```python
from build123d import *
from OCP.BRepFilletAPI import BRepFilletAPI_MakeChamfer

# Parameters (mm, degrees)
SKETCH_1_W          = 8
SKETCH_1_H          = 1
SKETCH_1_H_2        = 1.8
EXTRUDE_1_DEPTH     = 5.7
FILLET_1_R          = 0.8
CHAMFER_1_SIZE      = 0.5
CHAMFER_1_SIZE2     = 1.37373871
SKETCH_2_W          = 4.700894011
SKETCH_2_H          = 0.61177093
CUT_EXTRUDE_1_DEPTH = 5


with BuildPart() as part:
    # Эскиз1 → Бобышка-Вытянуть1 (new body)
    with BuildSketch(Plane.XY):
        with Locations((-3.289153283, 2.3)):
            Rectangle(SKETCH_1_W, SKETCH_1_H)
        with Locations((-3.289153283, 0.9)):
            Rectangle(SKETCH_1_W, SKETCH_1_H_2)
    extrude(amount=EXTRUDE_1_DEPTH)

    # Скругление1
    fillet_1_edges = [part.edges().sort_by_distance(p)[0] for p in [
        (0.710846717, 2.8, 2.85),
        (-7.289153283, 2.8, 2.85),
    ]]
    fillet(fillet_1_edges, radius=FILLET_1_R)

    # Фаска1: one chamfer whose edges measure the first distance from different faces: ONE call of the kernel's chamfer builder (chamfer() names one face for all edges)
    chamfer_1_edges_1 = [part.edges().sort_by_distance(p)[0] for p in [
        (0.710846717, 0, 2.85),
    ]]
    chamfer_1_side_1 = [part.faces().sort_by_distance(p)[0] for p in [
        (0.710846717, 1, 2.85),
    ]]
    chamfer_1_edges_2 = [part.edges().sort_by_distance(p)[0] for p in [
        (-7.289153283, 0, 2.85),
    ]]
    chamfer_1_side_2 = [part.faces().sort_by_distance(p)[0] for p in [
        (-7.289153283, 1, 2.85),
    ]]
    chamfer_1 = BRepFilletAPI_MakeChamfer(part.part.solid().wrapped)
    for e in chamfer_1_edges_1:
        chamfer_1.Add(CHAMFER_1_SIZE, CHAMFER_1_SIZE2, e.wrapped, chamfer_1_side_1[0].wrapped)  # the first distance lies on this face
    for e in chamfer_1_edges_2:
        chamfer_1.Add(CHAMFER_1_SIZE, CHAMFER_1_SIZE2, e.wrapped, chamfer_1_side_2[0].wrapped)  # the first distance lies on this face
    add(Compound.cast(chamfer_1.Shape()), mode=Mode.REPLACE)

    # Эскиз2 → Вырез-Вытянуть1 (cut)
    with BuildSketch(Plane(origin=(0, 0, 0), x_dir=(-1, 0, 0), z_dir=(0, 0, -1))):
        with BuildLine():
            Line((-0.310846717, 2), (-0.310846717, 0.780083015))
            Line((-0.310846717, 0.780083015), (0.733422785, 0.4))
            Line((0.733422785, 0.4), (5.844883781, 0.4))
            Line((5.844883781, 0.4), (6.889153283, 0.780083015))
            Line((6.889153283, 0.780083015), (6.889153283, 2))
            ThreePointArc((6.889153283, 2), (6.771995996, 2.282842712), (6.489153283, 2.4))
            Line((6.489153283, 2.4), (0.089153283, 2.4))
            ThreePointArc((0.089153283, 2.4), (-0.193689429, 2.282842712), (-0.310846717, 2))
        make_face()
        with Locations((3.494436776, 1.42533527)):
            Rectangle(SKETCH_2_W, SKETCH_2_H, mode=Mode.SUBTRACT)
    extrude(amount=-CUT_EXTRUDE_1_DEPTH, mode=Mode.SUBTRACT)


solid = part.part
```
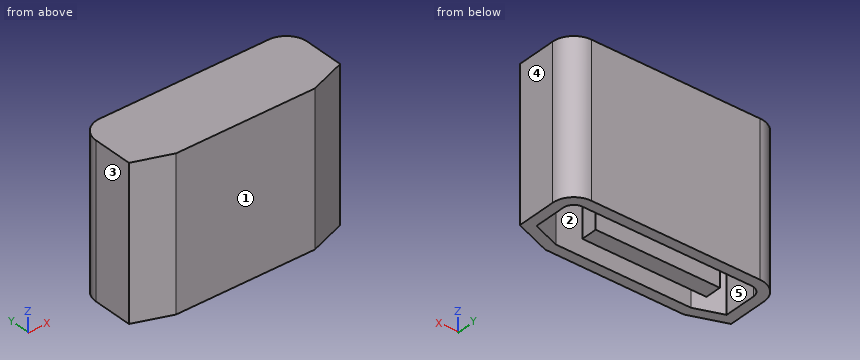
Input: part model. Units: mm. Frame: model coordinates. Face numbers are marked on the shaded views. A direction names the side the tool comes from. Round coordinates to 2 decimals unless told otherwise and drop trailing zeros. Order: outer loops, then holes, each group sorted by start corner. A loop starts at its lowest first (then second) coordinate and runs counter-clockwise, first axis right, second up. Notation, with made-up numbers: (-22.75, 84) - (31.25, 84) arc R12 cw to (31.25, 89) - close; hole circle Ø10 at (-4, 61). An arc over 180 degrees is marked (long way). Answer in a Markdown table with one row per item.
Item 1: Section query D-D (y = 1.55). Return the cut outline in (x, z).
Model answer:
| item | result |
|---|---|
| outline | (-7.29, 0) - (-6.89, 0) - (-6.89, 5) - (-5.84, 5) - (-5.84, 0) - (-1.14, 0) - (-1.14, 5) - (0.31, 5) - (0.31, 0) - (0.71, 0) - (0.71, 5.7) - (-7.29, 5.7) - close |
Item 2: Line query: line 1 (X direction, y = 1.6, z = 4.35); line 2 (Y direction, x = -3, z = 4.4); line 3 (X direction, y = 1.85, z = 0.8). Output: solid intervals per line, ascending.
Model answer:
| item | result |
|---|---|
| line 1 | x = -7.29 to -6.89, -5.84 to -1.14, 0.31 to 0.71 |
| line 2 | y = 0 to 0.4, 1.12 to 1.73, 2.4 to 2.8 |
| line 3 | x = -7.29 to -6.89, 0.31 to 0.71 |
Item 3: Section query C-C (x = -3.75). Return the cut outline in (y, z), then the cut area to 3 significant figures.
Model answer:
| item | result |
|---|---|
| outline | (0, 0) - (0.4, 0) - (0.4, 5) - (1.12, 5) - (1.12, 0) - (1.73, 0) - (1.73, 5) - (2.4, 5) - (2.4, 0) - (2.8, 0) - (2.8, 5.7) - (0, 5.7) - close |
| area | 9.02 mm² |
Item 4: Reachability of the marked faces 4 and 5 from +Z, -Z, +X, -X, +Y, -Y: full face, straight path, thin tool, end or side. Return the list, or none.
Model answer:
| item | result |
|---|---|
| face 4 | +Z, -Z, +X, +Y, -Y |
| face 5 | -Z |
Item 5: Section query B-B (y = 0.9). Return the cut outline in (x, z).
Model answer:
| item | result |
|---|---|
| outline | (-7.29, 0) - (-6.89, 0) - (-6.89, 5) - (0.31, 5) - (0.31, 0) - (0.71, 0) - (0.71, 5.7) - (-7.29, 5.7) - close |
Item 6: Section query A-A (z = 4.05). Return the cut outline in (x, y), then the cut area to 3 significant figures.
Model answer:
| item | result |
|---|---|
| outline | (-7.29, 0.5) - (-5.92, 0) - (-0.66, 0) - (0.71, 0.5) - (0.71, 2) arc R0.8 ccw to (-0.09, 2.8) - (-6.49, 2.8) arc R0.8 ccw to (-7.29, 2) - close; (-5.84, 1.12) - (-1.14, 1.12) - (-1.14, 1.73) - (-5.84, 1.73) - close; hole (-6.89, 0.78) - (-5.84, 0.4) - (-0.73, 0.4) - (0.31, 0.78) - (0.31, 2) arc R0.4 ccw to (-0.09, 2.4) - (-6.49, 2.4) arc R0.4 ccw to (-6.89, 2) - close |
| area | 10.4 mm² |
Item 7: Pin query (flat end, axial travel): pin 1 (1.5 mm diameter, centred on x = 0, z = 1.5, fed in from +Y). Return the tip coordinate at first contact, or that it passes through.
Model answer:
| item | result |
|---|---|
| pin 1 | stops at y = 2.8 |
Item 8: Mould query, pull axis Y, two halves, no side actions, for the marked faces 1, 2 and 3. Classes: released by +Y, released by -Y, zero draft, split by the parting line, or undercut.
Model answer:
| item | result |
|---|---|
| face 1 | released by -Y |
| face 2 | undercut |
| face 3 | zero draft |
